Autodesk Inventor part; units mm, degrees
ref_plane "YZ Plane" through (0, 0, 0) normal (1, 0, 0) x (0, 1, 0)
ref_plane "XZ Plane" through (0, 0, 0) normal (0, 1, 0) x (-1, 0, 0)
ref_plane "XY Plane" through (0, 0, 0) normal (0, 0, 1) x (1, 0, 0)
sketch "Sketch1" plane through (0, 0, 0) normal (0, 1, 0) x (-1, 0, 0)
  point P0 (0, 0)
sketch "Sketch2" plane through (0, 0, 0) normal (0, 1, 0) x (-1, 0, 0)
  line L0 (-12.7, 12.7) -> (12.7, 12.7)
  line L1 (12.7, 12.7) -> (12.7, -12.7)
  line L2 (12.7, -12.7) -> (-12.7, -12.7)
  line L3 (-12.7, -12.7) -> (-12.7, 12.7)
  line L4 (-12.7, 12.7) -> (12.7, -12.7) construction
  line L5 (12.7, 12.7) -> (-12.7, -12.7) construction
  line L6 (3.175, -15.24) -> (-3.175, -15.24)
  line L7 (-3.175, -15.24) -> (-3.175, -16.51)
  line L8 (-3.175, -16.51) -> (3.175, -16.51)
  line L9 (3.175, -16.51) -> (3.175, -15.24)
  line L10 (3.175, -15.24) -> (-3.175, -16.51) construction
  line L11 (-3.175, -15.24) -> (3.175, -16.51) construction
  line L12 (-1.27, -15.24) -> (1.27, -15.24)
  line L13 (1.27, -15.24) -> (1.27, -12.7)
  line L14 (1.27, -12.7) -> (-1.27, -12.7)
  line L15 (-1.27, -12.7) -> (-1.27, -15.24)
  line L16 (15.24, 3.175) -> (15.24, -3.175)
  line L17 (15.24, -3.175) -> (16.51, -3.175)
  line L18 (16.51, -3.175) -> (16.51, 3.175)
  line L19 (16.51, 3.175) -> (15.24, 3.175)
  line L20 (15.24, 3.175) -> (16.51, -3.175) construction
  line L21 (15.24, -3.175) -> (16.51, 3.175) construction
  line L22 (15.24, 1.27) -> (12.7, 1.27)
  line L23 (12.7, -1.27) -> (15.24, -1.27)
  line L24 (12.7, 1.27) -> (12.7, -1.27)
  line L25 (3.175, 10.16) -> (-3.175, 10.16)
  line L26 (-3.175, 10.16) -> (-3.175, 8.89)
  line L27 (-3.175, 8.89) -> (3.175, 8.89)
  line L28 (3.175, 8.89) -> (3.175, 10.16)
  line L29 (3.175, 10.16) -> (-3.175, 8.89) construction
  line L30 (-3.175, 10.16) -> (3.175, 8.89) construction
  line L31 (-1.27, 10.16) -> (1.27, 10.16)
  line L32 (1.27, 10.16) -> (1.27, 12.7)
  line L33 (1.27, 12.7) -> (-1.27, 12.7)
  line L34 (-1.27, 12.7) -> (-1.27, 10.16)
  line L35 (-8.89, 3.175) -> (-10.16, 3.175)
  line L36 (-10.16, -1.27) -> (-10.16, 1.27)
  line L37 (-10.16, -3.175) -> (-8.89, 3.175) construction
  line L38 (-10.16, -3.175) -> (-8.89, -3.175)
  line L39 (-10.16, 3.175) -> (-10.16, -3.175)
  line L40 (-8.89, -3.175) -> (-8.89, 3.175)
  line L41 (-10.16, 3.175) -> (-8.89, -3.175) construction
  line L42 (-10.16, 1.27) -> (-12.7, 1.27)
  line L43 (-12.7, 1.27) -> (-12.7, -1.27)
  line L44 (-12.7, -1.27) -> (-10.16, -1.27)
  point P0 (0, 0)
  point P1 (0, -15.875)
  point P2 (15.875, 0)
  point P3 (0, 9.525)
  point P4 (-9.525, 0)
  point P5 (-1.27, 12.7)
  point P6 (-10.16, 1.27)
  point P7 (-12.7, -1.27)
  point P8 (-1.27, -12.7)
  point P9 (1.27, -15.24)
  dimension "d0" = 25.4
  dimension "d1" = 25.4
  dimension "d16" = 6.35
  dimension "d17" = 1.27
  dimension "d18" = 2.54
  dimension "d19" = 2.54
  dimension "d20" = 1.27
  dimension "d23" = 90
  dimension "d25" = 6.35
  dimension "d26" = 1.27
  dimension "d27" = 2.54
  dimension "d28" = 1.27
  dimension "d29" = 2.54
  dimension "d32" = 90
extrude "Extrusion1" add sketch "Sketch2" along normal blind 9.525 contours L0 L34 L25 L26 L27 L28 L32 L1 L2 L3 L44 L39 L38 L40 L35 L42 | L0 L32 L25 L34 | L42 L36 L44 L3 | L25 L28 L27 L26 | L39 L35 L40 L38 L36
sketch "Sketch3" plane through (-12.7, 0, 12.7) normal (0, 0, 1) x (1, 0, 0)
  point P0 (12.7, 0)
sketch "Sketch4" plane through (-12.7, 0, 12.7) normal (0, 0, 1) x (1, 0, 0)
  line L0 (0, 9.525) -> (25.4, 9.525)
  line L1 (12.7, 0) -> (12.7, 9.525) construction
  line L2 (12.7, 6.35) -> (7.62, 6.35)
  line L3 (7.62, 6.35) -> (2.54, 9.525)
  line L4 (25.4, 9.525) -> (0, 9.525)
  line L5 (0, 0) -> (25.4, 0)
  line L6 (12.7, 6.35) -> (17.78, 6.35)
  line L7 (17.78, 6.35) -> (22.86, 9.525)
  point P0 (22.86, 9.525)
  dimension "d4" = 2.54
  dimension "d5" = 10.16
  dimension "d6" = 6.35
extrude "Extrusion2" cut sketch "Sketch4" against normal through all
pattern_circular "Circular Pattern1" count 2 over 90 about axis through (0, -10, 0) along (0, 1, 0) of "Extrusion2"
sketch "Sketch5" plane through (-5.08, 6.35, 12.7) normal (0, 1, 0) x (1, 0, 0)
  point P0 (5.08, 12.7)
sketch "Sketch6" plane through (0, 9.525, 0) normal (0, 1, 0) x (1, 0, 0)
  line L0 (11.1125, -11.1125) -> (-11.1125, -11.1125)
  line L1 (-11.1125, -11.1125) -> (-11.1125, 11.1125)
  line L2 (-11.1125, 11.1125) -> (11.1125, 11.1125)
  line L3 (11.1125, 11.1125) -> (11.1125, -11.1125)
  line L4 (11.1125, -11.1125) -> (-11.1125, 11.1125) construction
  line L5 (-11.1125, -11.1125) -> (11.1125, 11.1125) construction
  point P0 (0, 0)
  dimension "d12" = 22.225
  dimension "d13" = 22.225
extrude "Extrusion3" cut sketch "Sketch6" against normal blind 6.35
properties part number "Checker square thin"
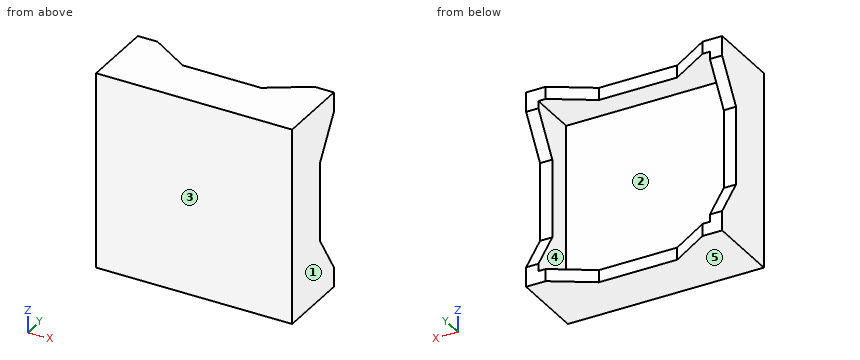
Model file for the job. Use its own axes, mm. Face numbers are marked on the shaded views. A direction names the side the tool comes from. Give positions to 0.01 mm unless a question says otherwise; leave off trailing zeros. Write each loop counter-clockwise with the first axis right and the second up, starting at its lowest first coordinate (ties: lowest second). Pieces come first, ordered by that corner, then holes. Notation, with made-up numbers: (17, 68.5) -> (27, 68.5) arc R18 ccw to (27, 72.5) -> close; hole circle Ø8 at (-29.5, 4). An arc over 180 degrees is marked (long way). Use CSV: the item, a comma, the result in double quotes. Start each with the question number.
1) Pin check, flat tips, straight feed: P1, Ø11, axis at x = -3.5, z = -2, coming from the +Y side (3 decimals); P2, Ø0.5, axis at x = -12, z = -1.5, coming from the +Y side. Stop position of each tip, or through.
2) Cut at B-B on y = 6. List the corners of the cut face in (x, z), plus the area to 3 significant figures.
3) Tool access for the marked faces 1 and 2: list every direction of +Z, -Z, +X, -X, +Y, -Y with a clear straight run to the whole face (end or side of a thin tool).
4) Cut at A-A on y = 8. List the corners of the cut face in (x, z).
5) Two-plate mould, pull along Z, no slides. Class the marked faces 3, 4 and 5: released by +Z, released by -Z, zero draft, split by the parting line, or undercut.
6) Drill centre lines: L1, parallel to Z at x = -3.5, y = 6; L2, parallel to Y at x = -5.25, z = 3.5 (3 decimals). Where is each one in solid material? Low to high.
Final values:
1,P1,"stops at y = 3.175"
1,P2,"stops at y = 6.35"
2,outline,"(-12.7, -12.7) -> (12.7, -12.7) -> (12.7, 12.7) -> (-12.7, 12.7) -> close; hole (-11.11, -11.11) -> (11.11, -11.11) -> (11.11, 11.11) -> (-11.11, 11.11) -> close"
2,area,"151 mm2"
3,face 1,"+Z, -Z, +X, +Y, -Y"
3,face 2,"+Y"
4,outline,"(-12.7, -12.7) -> (-7.72, -12.7) -> (-7.72, -11.11) -> (-11.11, -11.11) -> (-11.11, -7.72) -> (-12.7, -7.72) -> close; (-12.7, 7.72) -> (-11.11, 7.72) -> (-11.11, 11.11) -> (-7.72, 11.11) -> (-7.72, 12.7) -> (-12.7, 12.7) -> close; (7.72, -12.7) -> (12.7, -12.7) -> (12.7, -7.72) -> (11.11, -7.72) -> (11.11, -11.11) -> (7.72, -11.11) -> close; (7.72, 11.11) -> (11.11, 11.11) -> (11.11, 7.72) -> (12.7, 7.72) -> (12.7, 12.7) -> (7.72, 12.7) -> close"
5,face 3,"zero draft"
5,face 4,"undercut"
5,face 5,"released by -Z"
6,L1,"z = -12.7 to -11.11, 11.11 to 12.7"
6,L2,"y = 0 to 3.175"
